The listing builds one solid part. Answer for the finished solid, in the listing's coordinates (mm). A direction names the side the tool comes from. Coordinates: 2 decimals unless noted, no trailing zeros. Loops run counter-clockwise (first coordinate to the right, second up) from the corner with the lowest first, then second, coordinate; pieces in that order, holes last. Notation, with made-up numbers: (27, 69) - (67, 69) arc R20 ccw to (67, 92) - close; hole circle Ø2 at (-34, 49). An arc over 180 degrees is marked (long way). One line per question, with ' | ' between items.
from build123d import *

# Parameters (mm, degrees)
F0_W           = 95.9071815014
F0_H           = 83.329193294
F1_DEPTH       = 25.4
F2_W           = 57.4744343758
F2_H           = 52.2336028516
F3_DEPTH       = 12.7
F4_R           = 12.7
F6_D           = 9.525
F6_CBORE_D     = 15.875
F6_CBORE_DEPTH = 9.525


# Not quite as in the source:
# - a length typed as a fraction of an inch, garbled in the dataset ("3 / 203.2 mm" for 3/8 in), is restored


with BuildPart() as f1:
    # F0 (on Top) → F1 (new body)
    with BuildSketch(Plane.XY):
        Rectangle(F0_W, F0_H)
    extrude(amount=-F1_DEPTH)

    # F2 (on face) → F3 (cut)
    with BuildSketch(Plane.XY):
        Rectangle(F2_W, F2_H)
    extrude(amount=-F3_DEPTH, mode=Mode.SUBTRACT)

    # F4
    f4_edges = [f1.edges().sort_by_distance(p)[0] for p in [
        (-28.737217, 26.116801, -6.35),
        (28.737217, 26.116801, -6.35),
        (-28.737217, -26.116801, -6.35),
        (28.737217, -26.116801, -6.35),
    ]]
    fillet(f4_edges, radius=F4_R)

    # F6 (through all)
    with Locations(Plane.XY):
        with Locations((-31.75, 32.4055403471), (31.75, 32.4055403471), (31.75, -31.0944596529), (-31.75, -31.9523103535)):
            CounterBoreHole(F6_D / 2, F6_CBORE_D / 2, F6_CBORE_DEPTH)


solid = f1.part
Item 1: Find section A-A, the plane x = -31.75. Write down the section's boundary in (y, z) (3 decimals), plus the area to 3 significant figures.
Taken from the geometry:
outline: (-41.665, -25.4) - (-36.715, -25.4) - (-36.715, -9.525) - (-39.89, -9.525) - (-39.89, 0) - (-41.665, 0) - close; (-27.19, -25.4) - (27.643, -25.4) - (27.643, -9.525) - (24.468, -9.525) - (24.468, 0) - (-24.015, 0) - (-24.015, -9.525) - (-27.19, -9.525) - close; (37.168, -25.4) - (41.665, -25.4) - (41.665, 0) - (40.343, 0) - (40.343, -9.525) - (37.168, -9.525) - close | area: 1,510 mm2
Item 2: Each of these flat-tipped pins is pushed along its axis until it touches: pin 1 Ø5 at (x, y) = (35, 29.5) entering from +Z (3 decimals); pin 2 Ø15.5 at (x, y) = (-2, 8) entering from +Z. Where does it stop, or does it pass through?
Taken from the geometry:
pin 1: stops at z = -9.525 | pin 2: stops at z = -12.7
Item 3: Find section C-C, the plane y = 7. Write down the section's boundary in (x, z), plus the area to 3 significant figures.
Taken from the geometry:
outline: (-47.95, -25.4) - (47.95, -25.4) - (47.95, 0) - (28.74, 0) - (28.74, -12.7) - (-28.74, -12.7) - (-28.74, 0) - (-47.95, 0) - close | area: 1,710 mm2
Item 4: Which of the six approach directions +Z, -Z, +X, -X, +Y, -Y give full straight-line access (tool end or side, diameter ignored) to faces 1 (the face through (30.717, 40.275, -4.696)), 2 (the face through (27.21, 33.84, -17.57))?
Taken from the geometry:
face 1: +Z | face 2: +Z, -Z
Item 5: Find section D-D, the plane y = -34.5. Write down the section's boundary in (x, z) (3 decimals), plus the area to 3 significant figures.
Taken from the geometry:
outline: (-47.954, -25.4) - (-35.774, -25.4) - (-35.774, -9.525) - (-39.268, -9.525) - (-39.268, 0) - (-47.954, 0) - close; (-27.726, -25.4) - (28.421, -25.4) - (28.421, -9.525) - (24.58, -9.525) - (24.58, 0) - (-24.232, 0) - (-24.232, -9.525) - (-27.726, -9.525) - close; (35.079, -25.4) - (47.954, -25.4) - (47.954, 0) - (38.92, 0) - (38.92, -9.525) - (35.079, -9.525) - close | area: 1,920 mm2
Item 6: Find section B-B, the plane z = -19.25. State how many separate pieces and enclosed holes the cut face has, plus the area to 3 significant figures.
Taken from the geometry:
separate pieces: 1 | enclosed holes: 4 | area: 7,710 mm2
Item 7: Find the intervals of material crossed by line 1 (Y direction, x = 31.75, z = -6.5); line 2 (Y direction, x = -31.75, z = -6.75); line 3 (X direction, y = -33, z = -6.5), in increasing order. Write a range as [from, to].
Taken from the geometry:
line 1: y = [-41.66, -39.03], [-23.16, 24.47], [40.34, 41.66] | line 2: y = [-41.66, -39.89], [-24.01, 24.47], [40.34, 41.66] | line 3: x = [-47.95, -39.62], [-23.88, 24.04], [39.46, 47.95]
Item 8: The mould has two halves that part along Y. Classify faces 3 (the face through (-1, 28, 0)), 4 (the face through (-1, 41.665, -13)), 5 (the face through (-24.918, 22.495, -6.439)): pulls with the +Y half, pulls with the -Y half, needs draft (parallel to the pull), parting line crosses it, or undercut.
Taken from the geometry:
face 3: needs draft | face 4: pulls with the +Y half | face 5: undercut
